Here's how the part is built. I have some questions about the finished solid (model axes, mm). A direction names the side the tool comes from. Coordinates: 2 decimals unless noted, no trailing zeros. Write each loop counter-clockwise with the first axis right and the second up, starting at its lowest first coordinate (ties: lowest second). Pieces come first, ordered by that corner, then holes. Notation, with made-up numbers: M 77.5,69.25 L 121.5,69.25 A22 cw 121.5,98.25 Z; hole C 60,45 d7. An arc over 180 degrees is marked long. Use a Markdown table: item, result.
```python
from build123d import *

# Parameters (mm, degrees)
F0_W     = 19.05
F0_H     = 19.05
F1_DEPTH = 19.05


# Not quite as in the source:
# - a feature names something its author has since deleted; it is built from what else it names


with BuildPart() as f1:
    # F0 (on Front) → F1 (new body)
    with BuildSketch(Plane.XZ):
        Polygon((312.9268772483, -147.6505908728), (-296.6731227517, -147.6505908728), (-315.7231227517, -147.6505908728), (-315.7231227517, -166.7005908728), (-296.6731227517, -166.7005908728), (-296.6731227517, -185.7505908728), (-315.7231227517, -185.7505908728), (-315.7231227517, -204.8005908728), (-296.6731227517, -204.8005908728), (312.9268772483, -204.8005908728), (312.9268772483, -185.7505908728), (312.9268772483, -166.7005908728), align=None)
        with Locations((322.4518772483, -157.1755908728)):
            Rectangle(F0_W, F0_H)
        with Locations((322.4518772483, -195.2755908728)):
            Rectangle(F0_W, F0_H)
    extrude(amount=F1_DEPTH)


solid = f1.part
```
1. Suppose I cut it at A-A on y = -15.5. Write out the boundary of the cut face in (x, z), and give its area (3 significant figures).
Answers follow:
| item | result |
|---|---|
| outline | M -315.72,-204.8 L 331.98,-204.8 L 331.98,-185.75 L 312.93,-185.75 L 312.93,-166.7 L 331.98,-166.7 L 331.98,-147.65 L -315.72,-147.65 L -315.72,-166.7 L -296.67,-166.7 L -296.67,-185.75 L -315.72,-185.75 Z |
| area | 36,300 mm2 |
2. Which directions (+Z, -Z, +X, -X, +Y, -Y) give clear straight access to the entire face, cutting with the end or side of a thin tool? Please do faces 1 (the face through (322, -9, -166.701)), 2 (the face through (-315.723, -9, -195)), 3 (the face through (-296.673, -9, -176)).
Answers follow:
| item | result |
|---|---|
| face 1 | +X, +Y, -Y |
| face 2 | +Z, -Z, -X, +Y, -Y |
| face 3 | -X, +Y, -Y |
3. I need wall thicknesses on probe 1 along X at (y, z) = (-2, -168.5). Which ranges of the line are inside material? Lowest first, please.
Answers follow:
| item | result |
|---|---|
| probe 1 | x = -296.67 to 312.93 |
4. We'd pull the mould along Z, two halves only. Please class faces 4 (the face through (4, -9, -204.801)), 5 (the face through (4, -19.05, -176)), 6 (the face through (322, -9, -185.751)): +Z half, -Z half, draft (parallel to the pull), parting line (faces both ways), or undercut.
Answers follow:
| item | result |
|---|---|
| face 4 | -Z half |
| face 5 | draft |
| face 6 | undercut |
5. Will this pin go through, and if not, where does the flat tip stop? pin 1 Ø1 at (y, z) = (-16, -182.5) entering from +X.
Answers follow:
| item | result |
|---|---|
| pin 1 | stops at x = 312.93 |
6. Suppose I cut it at B-B on z = -174.5. Write out the boundary of the cut face in (x, y), and give its area (3 significant figures).
Answers follow:
| item | result |
|---|---|
| outline | M -296.67,-19.05 L 312.93,-19.05 L 312.93,0 L -296.67,0 Z |
| area | 11,600 mm2 |
